from build123d import *

# Parameters (mm, degrees)
BOSS_EXTRUDE1_DEPTH = 5


with BuildPart() as part:
    # Sketch1 → Boss-Extrude1 (new body)
    with BuildSketch(Plane(origin=(0, 0, 0), x_dir=(1, 0, 0), z_dir=(0, 1, 0))):
        Polygon((-72.763800855, -36.482591992), (-67.763800855, -36.482591992), (-67.763800855, -42.832591992), (-52.763800855, -42.832591992), (-52.763800855, -36.482591992), (-47.763800855, -36.482591992), (-47.763800855, -1.40972798), (-13.434360787, 17.088978271), (20.89507928, -1.40972798), (20.89507928, -36.482591992), (25.89507928, -36.482591992), (25.89507928, -42.832591992), (40.89507928, -42.832591992), (40.89507928, -36.482591992), (45.89507928, -36.482591992), (45.89507928, 13.517408008), (-10.934360787, 42.661627557), (-10.934360787, 23.003270856), (-15.934360787, 23.003270856), (-15.934360787, 44.14042767), (-72.763800855, 13.517408008), align=None)
    extrude(amount=BOSS_EXTRUDE1_DEPTH)


solid = part.part
The listing builds one solid part. Answer for the finished solid, in the listing's coordinates (mm). A direction names the side the tool comes from. Coordinates: 2 decimals unless noted, no trailing zeros. Write each loop counter-clockwise with the first axis right and the second up, starting at its lowest first coordinate (ties: lowest second). Pieces come first, ordered by that corner, then holes. Notation, with made-up numbers: M 13.5,11.25 L 55.5,11.25 A13 ccw 55.5,23.25 Z; hole C 32.5,17 d6. An arc over 180 degrees is marked long. Write each question's results on one line, items separated by ' | '.
Item 1: The part is cut by section A-A on z = -32. Determine the outline of the cut face in (x, y), and give its area (3 significant figures).
Answer below:
outline: M -38.46,0 L -15.93,0 L -15.93,5 L -38.46,5 Z; M -10.93,0 L 9.86,0 L 9.86,5 L -10.93,5 Z | area: 217 mm2
Item 2: The part is cut by section C-C on z = 8.5. Determine the outline of the cut face in (x, y), and give its area (3 significant figures).
Answer below:
outline: M -72.76,0 L -47.76,0 L -47.76,5 L -72.76,5 Z; M 20.9,0 L 45.9,0 L 45.9,5 L 20.9,5 Z | area: 250 mm2
Item 3: Given P1, Ø1.5, axis at x = -49.5, y = 2, coming from the +Z side; P2, Ø2.5, axis at y = 1.5, z = 38.5, coming from the +X side; P3, Ø2.5, axis at x = -14, y = 3.5, coming from the -Z side, each flat-ended and moving along its own axis, determine where each tip first touches the part or whether it passes through.
Answer below:
P1: z = 36.48 | P2: x = 40.9 | P3: z = -23
Item 4: The part is cut by section D-D on x = 19.5. Determine the outline of the cut face in (y, z).
Answer below:
outline: M 0,-27.05 L 5,-27.05 L 5,0.66 L 0,0.66 Z
Item 5: Which of the six approach directions +Z, -Z, +X, -X, +Y, -Y give full straight-line access (tool end or side, diameter ignored) to faces 1 (the face through (20.895, 2, 19)), 2 (the face through (40.895, 2, 40)), 3 (the face through (-10.934, 2, -33)), 4 (the face through (45.895, 2, 12)), 5 (the face through (-70, 2, 36.483))?
Answer below:
face 1: +Z, +Y, -Y | face 2: +Z, +X, +Y, -Y | face 3: -Z, +Y, -Y | face 4: +Z, -Z, +X, +Y, -Y | face 5: +Z, -X, +Y, -Y
Item 6: Consider probe 1 along X at (y, z) = (3, 5); probe 2 along X at (y, z) = (3.9, -16); probe 3 along Z at (x, y) = (-51, 2.1). Determine where each line is inside the solid, lowest interval first. Write a range as [from, to].
Answer below:
probe 1: [-72.76, -47.76], [20.9, 45.9] | probe 2: [-68.16, -15.46], [-11.41, 41.05] | probe 3: [-25.25, 36.48]
Item 7: The part is cut by section B-B on y = 2.95. Determine the outline of the cut face in (x, z), and give its area (3 significant figures).
Answer below:
outline: M -72.76,-13.52 L -15.93,-44.14 L -15.93,-23 L -10.93,-23 L -10.93,-42.66 L 45.9,-13.52 L 45.9,36.48 L 40.9,36.48 L 40.9,42.83 L 25.9,42.83 L 25.9,36.48 L 20.9,36.48 L 20.9,1.41 L -13.43,-17.09 L -47.76,1.41 L -47.76,36.48 L -52.76,36.48 L -52.76,42.83 L -67.76,42.83 L -67.76,36.48 L -72.76,36.48 Z | area: 4,830 mm2
